Answer from the drawing. Dimensions are ordinates in mm from the lowest x, y and z of the part. Round coordinates to 2 decimals unless told otherwise and drop trailing zeros. Loops run counter-clockwise (first coordinate to the right, second up) from the corner with the lowest first, then second, coordinate; pieces in that order, holes last. Notation, with made-up numbers: (0, 44) - (50, 44) arc R12 cw to (50, 59) - close; hole circle Ø4 at (-15, 51.5). An arc over 180 degrees is marked (long way). Use CSV: the item, a comma, the result in double quotes. Start each with the question number.
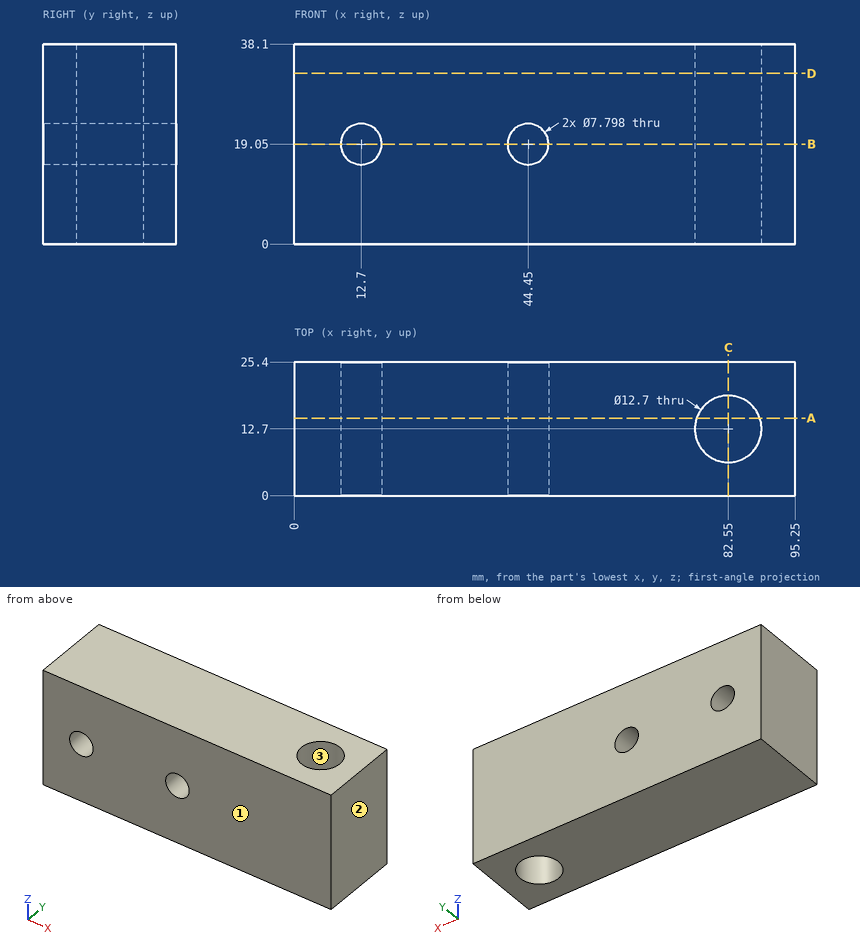
Item 1: A cutting plane is placed at C-C (x = 82.55). Determine the outline of the cut face in (y, z), plus the area to 3 significant figures.
Item 2: The mould has two halves that part along X. Classify the marked faces 1, 2 and 3: pulls with the +X half, pulls with the -X half, needs draft (parallel to the pull), parting line crosses it, or undercut.
Item 3: Find the intervals of material crossed by probe 1 along X at (y, z) = (20, 19.05); probe 2 along Z at (x, y) = (44.45, 9.25); probe 3 along X at (y, z) = (21.25, 20), in increasing order. Write a range as [from, to].
Item 4: A cutting plane is placed at A-A (y = 14.75). Determine the outline of the cut face in (x, z), plus the area to 3 significant figures.
Item 5: A cutting plane is placed at B-B (z = 19.05). Determine the outline of the cut face in (x, y).
Item 6: A cutting plane is placed at D-D (z = 32.5). Determine the outline of the cut face in (x, y).
Result sheet:
1,outline,"(0, 0) - (6.35, 0) - (6.35, 38.1) - (0, 38.1) - close; (19.05, 0) - (25.4, 0) - (25.4, 38.1) - (19.05, 38.1) - close"
1,area,"484 mm^2"
2,face 1,"needs draft"
2,face 2,"pulls with the +X half"
2,face 3,"undercut"
3,probe 1,"[0, 8.8], [16.6, 40.55], [48.35, 95.25]"
3,probe 2,"[0, 15.15], [22.95, 38.1]"
3,probe 3,"[0, 8.92], [16.48, 40.67], [48.23, 95.25]"
4,outline,"(0, 0) - (76.54, 0) - (76.54, 38.1) - (0, 38.1) - close; (88.56, 0) - (95.25, 0) - (95.25, 38.1) - (88.56, 38.1) - close; hole circle Ø7.8 at (12.7, 19.05); hole circle Ø7.8 at (44.45, 19.05)"
4,area,"3,080 mm^2"
5,outline,"(0, 0) - (8.8, 0) - (8.8, 25.4) - (0, 25.4) - close; (16.6, 0) - (40.55, 0) - (40.55, 25.4) - (16.6, 25.4) - close; (48.35, 0) - (95.25, 0) - (95.25, 25.4) - (48.35, 25.4) - close; hole circle Ø12.7 at (82.55, 12.7)"
6,outline,"(0, 0) - (95.25, 0) - (95.25, 25.4) - (0, 25.4) - close; hole circle Ø12.7 at (82.55, 12.7)"
